from build123d import *

# Parameters (mm, degrees)
SKETCH1_R           = 5.57
BOSS_EXTRUDE1_DEPTH = 44
CHAMFER1_SIZE       = 17
CHAMFER1_SIZE2      = 5
SKETCH2_R           = 8.25
BOSS_EXTRUDE2_DEPTH = 2


with BuildPart() as part:
    # Sketch1 → Boss-Extrude1 (new body)
    with BuildSketch(Plane(origin=(0, 0, 0), x_dir=(1, 0, 0), z_dir=(0, 1, 0))):
        with Locations(Location((0, 0, 0), (0, 0, 270))):
            Circle(SKETCH1_R)
    extrude(amount=BOSS_EXTRUDE1_DEPTH)

    # Chamfer1
    chamfer1_edges = [part.edges().sort_by_distance(p)[0] for p in [
        (0, 44, -5.57),
    ]]
    chamfer1_side = [part.faces().sort_by_distance(p)[0] for p in [
        (0, 22, -5.57),
    ]]
    chamfer(chamfer1_edges, length=CHAMFER1_SIZE, length2=CHAMFER1_SIZE2, reference=chamfer1_side[0])

    # Sketch2 → Boss-Extrude2 (add)
    with BuildSketch(Plane(origin=(0, 16, 0), x_dir=(1, 0, 0), z_dir=(0, 1, 0))):
        with Locations(Location((0, 0, 0), (0, 0, 270))):
            Circle(SKETCH2_R)
    extrude(amount=-BOSS_EXTRUDE2_DEPTH)


solid = part.part
The listing builds one solid part. Answer for the finished solid, in the listing's coordinates (mm). A direction names the side the tool comes from. Coordinates: 2 decimals unless noted, no trailing zeros. Write each loop counter-clockwise with the first axis right and the second up, starting at its lowest first coordinate (ties: lowest second). Pieces come first, ordered by that corner, then holes. Notation, with made-up numbers: (55.5, 21) -> (69.5, 21) arc R20 cw to (69.5, 53) -> close; hole circle Ø3 at (42.25, 12). An arc over 180 degrees is marked (long way). One line per question, with ' | ' between items.
1. Section D-D (z = 6.5) is taken. Determine the outline of the cut face in (x, y), and give its area (3 significant figures).
Verdict:
outline: (-5.08, 14) -> (5.08, 14) -> (5.08, 16) -> (-5.08, 16) -> close | area: 20.3 mm^2
2. Section A-A (z = 0) is taken. Determine the outline of the cut face in (x, y).
Verdict:
outline: (-8.25, 14) -> (-5.57, 14) -> (-5.57, 0) -> (5.57, 0) -> (5.57, 14) -> (8.25, 14) -> (8.25, 16) -> (5.57, 16) -> (5.57, 27) -> (0.57, 44) -> (-0.57, 44) -> (-5.57, 27) -> (-5.57, 16) -> (-8.25, 16) -> close
3. Section C-C (y = 37) is taken. Determine the outline of the cut face in (x, z).
Verdict:
outline: circle Ø5.26 at (0, 0)
4. Straight lines are drawn through the part: line 1 (X direction, y = 9.5, z = 0); line 2 (Y direction, x = -3.25, z = 5.5); line 3 (Z direction, x = -2.5, y = 5.5). For each, find the intervals that lie inside material, in ascending order.
Verdict:
line 1: x = -5.57 to 5.57 | line 2: y = 14 to 16 | line 3: z = -4.98 to 4.98
5. Given pin 1 Ø5 at (x, z) = (3.5, -4.5) entering from -Y; pin 2 Ø5 at (x, y) = (4.5, 7) entering from +Z; pin 3 Ø5 at (y, z) = (33, 2) entering from -X; pin 4 Ø2 at (y, z) = (21, -4.5) entering from -X, each flat-ended and moving along its own axis, determine where each tip first touches the part or whether it passes through.
Verdict:
pin 1: stops at y = 0 | pin 2: stops at z = 5.2 | pin 3: stops at x = -4.38 | pin 4: stops at x = -4.33
6. Which of the six approach directions +Z, -Z, +X, -X, +Y, -Y give full straight-line access (tool end or side, diameter ignored) to faces 1 (the cylindrical face through (-5.438, 6.902, -1.207)), 2 (the flat face through (1.9, 16, 5.4)), 3 (the flat face through (0, 0, 0))?
Verdict:
face 1: -Y | face 2: +Y | face 3: +Z, -Z, +X, -X, -Y
7. Section B-B (y = 5) is taken. Determine the outline of the cut face in (x, z).
Verdict:
outline: circle Ø11.14 at (0, 0)
